```python
from build123d import *

# Parameters (mm, degrees)
CROQUIS1_W              = 120
CROQUIS1_H              = 60
CROQUIS1_R              = 10
SALIENTE_EXTRUIR1_DEPTH = 15
CROQUIS2_W              = 35
CROQUIS2_H              = 25
SALIENTE_EXTRUIR2_DEPTH = 10


with BuildPart() as part:
    # Croquis1 → Saliente-Extruir1 (new body)
    with BuildSketch(Plane(origin=(0, 0, 0), x_dir=(1, 0, 0), z_dir=(0, 1, 0))):
        Rectangle(CROQUIS1_W, CROQUIS1_H)
        with Locations(Location((40, -10, 0), (0, 0, 270))):
            Circle(CROQUIS1_R, mode=Mode.SUBTRACT)
    extrude(amount=SALIENTE_EXTRUIR1_DEPTH)

    # Croquis2 → Saliente-Extruir2 (add)
    with BuildSketch(Plane(origin=(0, 15, 0), x_dir=(1, 0, 0), z_dir=(0, 1, 0))):
        with Locations((-42.5, 17.5)):
            Rectangle(CROQUIS2_W, CROQUIS2_H)
    extrude(amount=SALIENTE_EXTRUIR2_DEPTH)


solid = part.part
```
For this review, take the finished solid that the model builds, in its own axes (mm). A direction names the side the tool comes from. Coordinates: 2 decimals unless noted, no trailing zeros. Write each loop counter-clockwise with the first axis right and the second up, starting at its lowest first coordinate (ties: lowest second). Pieces come first, ordered by that corner, then holes. Notation, with made-up numbers: (82, 0.5) - (89, 0.5) arc R25 cw to (89, 33.5) - close; hole circle Ø2 at (45.5, -27.5). An arc over 180 degrees is marked (long way). Put each result on its own line as item: value.
1. Add section B-B, the plane x = 40. Give the boundary of the cut face in (y, z).
Values found:
outline: (0, -30) - (15, -30) - (15, 0) - (0, 0) - close; (0, 20) - (15, 20) - (15, 30) - (0, 30) - close
2. Wall thickness on probe 1 along X at (y, z) = (9.5, 10); probe 2 along Y at (x, z) = (54, -23); probe 3 along X at (y, z) = (23.5, -8.5): over which ranges is each line inside the solid? List them lowest first.
Values found:
probe 1: -60 to 30, 50 to 60
probe 2: 0 to 15
probe 3: -60 to -25
3. Mouldability with a two-part tool opening along X and no side actions: class faces 1 (the flat face through (60, 7, 0)), 2 (the cylindrical face through (30.24, 7.4, 7.83)), 3 (the flat face through (-60, 10, -6)), 4 (the flat face through (-1, 7, 30)) as released by +X, released by -X, zero draft, split by the parting line, or undercut.
Values found:
face 1: released by +X
face 2: undercut
face 3: released by -X
face 4: zero draft
4. Add section D-D, the plane x = -47.5. Give the boundary of the cut face in (y, z), then the cut area to 3 significant figures.
Values found:
outline: (0, -30) - (25, -30) - (25, -5) - (15, -5) - (15, 30) - (0, 30) - close
area: 1,150 mm²
5. For pin 1 (5 mm diameter, centred on x = -42.5, y = 20.5, fed in from +Z), flat-tipped, find the tip position at first contact; note if it passes through.
Values found:
pin 1: z = -5
6. Add section A-A, the plane z = 10. Give the boundary of the cut face in (x, y).
Values found:
outline: (-60, 0) - (30, 0) - (30, 15) - (-60, 15) - close; (50, 0) - (60, 0) - (60, 15) - (50, 15) - close
7. Machinability: for faces 5 (the flat face through (-43, 25, -18)), 6 (the flat face through (-43, 20, -5)), 7 (the flat face through (-25, 20, -17)), which of the approach directions +Z, -Z, +X, -X, +Y, -Y give a long, thin tool a straight path to every point of the face, cutting with its end or side? Answer none if there is none.
Values found:
face 5: +Z, -Z, +X, -X, +Y
face 6: +Z, +X, -X, +Y
face 7: +Z, -Z, +X, +Y
8. Add section C-C, the plane y = 2.75. Give the boundary of the cut face in (x, z), then the cut area to 3 significant figures.
Values found:
outline: (-60, -30) - (60, -30) - (60, 30) - (-60, 30) - close; hole circle Ø20 at (40, 10)
area: 6,890 mm²
